Geometry check sheet. Reference: the model listing, model coordinates, mm. Coordinates: 2 decimals unless noted, no trailing zeros. Write each loop counter-clockwise with the first axis right and the second up, starting at its lowest first coordinate (ties: lowest second). Pieces come first, ordered by that corner, then holes.
from build123d import *

# Parameters (mm, degrees)
SKETCH1_R           = 2.25
SKETCH1_R_2         = 0.8
SKETCH1_R_3         = 1.7526
BOSS_EXTRUDE1_DEPTH = 3.1115


with BuildPart() as part:
    # Sketch1 → Boss-Extrude1 (new body)
    with BuildSketch(Plane.XY):
        with BuildLine():
            Line((40.571674968, -45.901211355), (107.95698504, 3.057082175))
            Line((107.95698504, 3.057082175), (114.431306158, 3.057082175))
            Line((114.431306158, 3.057082175), (129.0733448, -17.095955091))
            add(Edge.make_bspline(
                [(129.0733448, -17.095955091), (133.53865967, -23.241933746), (138.918061624, -28.349297229), (145.211550663, -32.41804554)],
                knots=[0.5, 0.5, 0.5, 0.5, 0.915854192, 0.915854192, 0.915854192, 0.915854192], degree=3))
            ThreePointArc((145.211550663, -32.41804554), (159.788231987, -36.343991717), (150.867180903, -24.165833426))
            Line((150.867180903, -24.165833426), (150.640762289, -24.020208846))
            add(Edge.make_bspline(
                [(137.163514743, -11.218102568), (137.631181225, -11.861790257), (138.599969423, -13.134624479), (140.611611711, -15.54248749), (143.29771775, -18.340403293), (146.787953317, -21.358895338), (149.334712498, -23.17584607), (150.640762289, -24.020208846)],
                knots=[0.5, 0.5, 0.5, 0.5, 0.551981774, 0.603963548, 0.707927096, 0.811890644, 0.915854192, 0.915854192, 0.915854192, 0.915854192], degree=3))
            Line((137.163514743, -11.218102568), (120.284653169, 12.013657342))
            Line((120.284653169, 12.013657342), (120.976190903, 12.516088915))
            Line((120.976190903, 12.516088915), (147.319477841, 31.655607203))
            Line((147.319477841, 31.655607203), (145.885321673, 33.629553824))
            Line((145.885321673, 33.629553824), (134.586350681, 49.181253217))
            ThreePointArc((134.586350681, 49.181253217), (131.845960487, 51.269897662), (128.408504904, 51.506695351))
            Line((128.408504904, 51.506695351), (106.294747249, 46.504613793))
            ThreePointArc((106.294747249, 46.504613793), (102.544365306, 43.854529448), (101.766337412, 39.328716333))
            Line((101.766337412, 39.328716333), (101.888205656, 38.789947666))
            ThreePointArc((101.888205656, 38.789947666), (102.771567105, 37.539820352), (104.280171476, 37.280477721))
            Line((104.280171476, 37.280477721), (124.755382254, 41.911923712))
            ThreePointArc((124.755382254, 41.911923712), (128.192837837, 41.675126022), (130.933228031, 39.586481577))
            Line((130.933228031, 39.586481577), (134.488040457, 34.693702023))
            Line((134.488040457, 34.693702023), (110.217530626, 17.060144455))
            Line((110.217530626, 17.060144455), (34.693822445, 17.060144455))
            Line((34.693822445, 17.060144455), (-20.306177555, 17.060144455))
            Line((-20.306177555, 17.060144455), (-20.306177555, 7.060144459))
            Line((-20.306177555, 7.060144459), (-20.306177555, 3.057082175))
            Line((-20.306177555, 3.057082175), (-1.445233082, 3.057082175))
            Line((-1.445233082, 3.057082175), (-19.142654999, -45.566184926))
            Line((-19.142654999, -45.566184926), (-8.82525124, -49.321412789))
            Line((-8.82525124, -49.321412789), (-8.82525124, -46.273412789))
            Line((-8.82525124, -46.273412789), (-2.94645984, -46.273412789))
            Line((-2.94645984, -46.273412789), (-2.94645984, -44.075412789))
            Line((-2.94645984, -44.075412789), (-5.14645984, -44.075412789))
            Line((-5.14645984, -44.075412789), (-5.14645984, -41.075412789))
            Line((-5.14645984, -41.075412789), (-2.94645984, -41.075412789))
            Line((-2.94645984, -41.075412789), (-2.94645984, -39.575412789))
            Line((-2.94645984, -39.575412789), (0.65354016, -39.575412789))
            Line((0.65354016, -39.575412789), (0.65354016, -41.075412789))
            Line((0.65354016, -41.075412789), (2.85354016, -41.075412789))
            Line((2.85354016, -41.075412789), (2.85354016, -44.075412789))
            Line((2.85354016, -44.075412789), (0.65354016, -44.075412789))
            Line((0.65354016, -44.075412789), (0.65354016, -46.273412789))
            Line((0.65354016, -46.273412789), (21.695957359, -46.273412789))
            Line((21.695957359, -46.273412789), (21.695957359, -44.075412789))
            Line((21.695957359, -44.075412789), (19.495957359, -44.075412789))
            Line((19.495957359, -44.075412789), (19.495957359, -41.075412789))
            Line((19.495957359, -41.075412789), (21.695957359, -41.075412789))
            Line((21.695957359, -41.075412789), (21.695957359, -39.575412789))
            Line((21.695957359, -39.575412789), (25.295957359, -39.575412789))
            Line((25.295957359, -39.575412789), (25.295957359, -41.075412789))
            Line((25.295957359, -41.075412789), (27.495957359, -41.075412789))
            Line((27.495957359, -41.075412789), (27.495957359, -44.075412789))
            Line((27.495957359, -44.075412789), (25.295957359, -44.075412789))
            Line((25.295957359, -44.075412789), (25.295957359, -46.273412789))
            Line((25.295957359, -46.273412789), (31.17474876, -46.273412789))
            Line((31.17474876, -46.273412789), (31.17474876, -49.321412789))
            Line((31.17474876, -49.321412789), (40.571674968, -45.901211355))
        make_face()
        with Locations((153.189271476, -31.821412789)):
            Circle(SKETCH1_R, mode=Mode.SUBTRACT)
        with Locations((156.829847951, -29.176379153)):
            Circle(SKETCH1_R_2, mode=Mode.SUBTRACT)
        with Locations((149.548695001, -34.466446424)):
            Circle(SKETCH1_R_2, mode=Mode.SUBTRACT)
        with Locations((-4.689464322, 6.397861115)):
            Circle(SKETCH1_R_3, mode=Mode.SUBTRACT)
        with Locations((28.910535678, 6.397861115)):
            Circle(SKETCH1_R_3, mode=Mode.SUBTRACT)
        Polygon((22.752313402, 3.057082175), (82.411954897, 3.057082175), (35.229290336, -31.223130213), align=None, mode=Mode.SUBTRACT)
        Polygon((24.587512611, -31.223130213), (12.110535678, 3.057082175), (9.196544643, 3.057082175), (-3.28043229, -31.223130213), align=None, mode=Mode.SUBTRACT)
        with BuildLine():
            Line((88.543835939, 13.524152696), (92.543835721, 13.522830074))
            ThreePointArc((92.543835721, 13.522830074), (94.043339655, 12.022334173), (92.542843754, 10.522830238))
            Line((92.542843754, 10.522830238), (88.542843973, 10.52415286))
            ThreePointArc((88.542843973, 10.52415286), (87.043340038, 12.024648761), (88.543835939, 13.524152696))
        make_face(mode=Mode.SUBTRACT)
        with BuildLine():
            Line((120.546853002, 5.529529102), (122.932016073, 2.318454963))
            ThreePointArc((122.932016073, 2.318454963), (122.622299423, 0.21986601), (120.523710469, 0.52958266))
            Line((120.523710469, 0.52958266), (118.138547398, 3.740656799))
            ThreePointArc((118.138547398, 3.740656799), (118.448264049, 5.839245752), (120.546853002, 5.529529102))
        make_face(mode=Mode.SUBTRACT)
        Polygon((131.942859267, -12.538994841), (130.401681893, -13.658725747), (129.514126162, -12.437110085), (132.59648091, -10.197648274), (133.484036641, -11.419263935), align=None, mode=Mode.SUBTRACT)
        Polygon((134.294000276, -15.775062818), (135.835177651, -14.655331913), (136.722733382, -15.876947574), (133.640378633, -18.116409385), (132.752822902, -16.894793724), align=None, mode=Mode.SUBTRACT)
        Polygon((138.289721592, 30.886083745), (139.177277323, 29.664468084), (142.259632072, 31.903929895), (141.372076341, 33.125545557), align=None, mode=Mode.SUBTRACT)
        Polygon((40.244952044, -40.34761098), (43.327306792, -38.108149169), (44.214862523, -39.32976483), (41.132507775, -41.569226641), align=None, mode=Mode.SUBTRACT)
        Polygon((134.024760687, 43.238257986), (132.483583313, 42.118527081), (131.596027582, 43.340142742), (134.67838233, 45.579604554), (135.565938061, 44.357988892), align=None, mode=Mode.SUBTRACT)
        Polygon((136.375901696, 40.002190009), (137.917079071, 41.121920915), (138.804634802, 39.900305253), (135.722280053, 37.660843442), (134.834724322, 38.882459103), align=None, mode=Mode.SUBTRACT)
        Polygon((6.110535678, 4.873861115), (18.110535678, 4.873861115), (18.110535678, 7.921861115), (12.110535678, 7.921861115), (6.110535678, 7.921861115), align=None, mode=Mode.SUBTRACT)
    extrude(amount=BOSS_EXTRUDE1_DEPTH)


solid = part.part
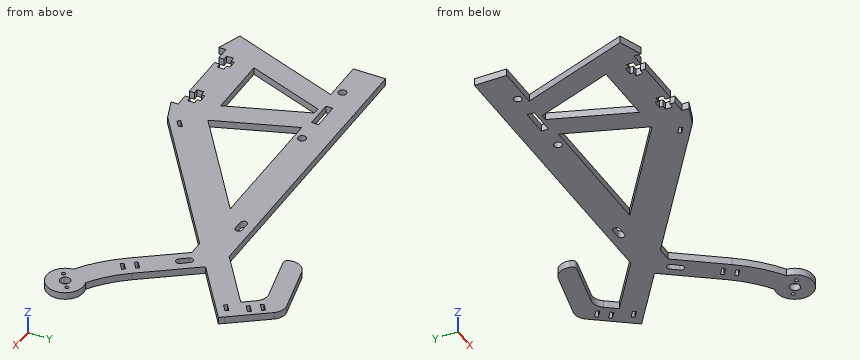
1. Gauge pin test, flat ends, axial feed: pin 1 Ø1.5 at (x, z) = (38.5, 0.5) entering from +Y; pin 2 Ø0.9 at (x, z) = (29.5, 1.5) entering from -Y; pin 3 Ø1.5 at (y, z) = (-43, 2) entering from +X. Record the tip position at first contact, or that the pin passes through.
Computed values:
pin 1: stops at y = 17.06
pin 2: stops at y = -46.27
pin 3: stops at x = 45.6
2. Thickness scan on line 1 along Y through (x, z) = (9.5, 2.85); line 2 along X through (y, z) = (6, 1); line 3 along X through (y, z) = (5, 1.3). Record the ranges inside material, lowest first.
Computed values:
line 1: y = -46.27 to -31.22, 3.06 to 4.87, 7.92 to 17.06
line 2: x = -20.31 to -6.4, -2.98 to 6.11, 18.11 to 27.2, 30.62 to 118.72, 119.96 to 124.65
line 3: x = -20.31 to -5.75, -3.63 to 6.11, 18.11 to 27.85, 29.97 to 117.89, 120.94 to 125.38
3. Sectioned sample at A-A, the plane y = -8. Record the boundary of the cut face in (x, z).
Computed values:
outline: (-5.47, 0) - (5.17, 0) - (5.17, 3.11) - (-5.47, 3.11) - close; (16.13, 0) - (26.78, 0) - (26.78, 3.11) - (16.13, 3.11) - close; (67.19, 0) - (92.74, 0) - (92.74, 3.11) - (67.19, 3.11) - close; (122.46, 0) - (134.83, 0) - (134.83, 3.11) - (122.46, 3.11) - close
4. Sectioned sample at B-B, the plane z = 0.5. Give the number of separate pieces and of enclosed holes in the cut face, and give its area (3 significant figures).
Computed values:
separate pieces: 1
enclosed holes: 16
area: 5,710 mm2
